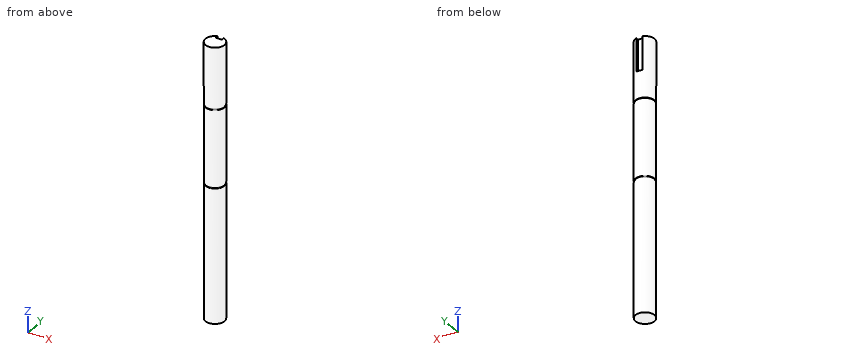
```python
from build123d import *

# Parameters (mm, degrees)
SKETCH_1_R          = 12.5
EXTRUDE_1_DEPTH     = 359
CUT_EXTRUDE_START   = -44
SKETCH_2_W          = 8
SKETCH_2_H          = 8.5
CUT_EXTRUDE_1_DEPTH = 44
SKETCH_3_W          = 1.4
SKETCH_3_H          = 2.395884976
SKETCH_3_H_2        = 2.262849939


with BuildPart() as part:
    # Эскиз1 → Бобышка-Вытянуть1 (new body)
    with BuildSketch(Plane.XY):
        Circle(SKETCH_1_R)
    extrude(amount=-EXTRUDE_1_DEPTH)

    # Эскиз2 → Вырез-Вытянуть1 (cut)
    with BuildSketch(Plane.XY.offset(CUT_EXTRUDE_START)):
        with Locations((0, 12.25)):
            Rectangle(SKETCH_2_W, SKETCH_2_H)
    extrude(amount=CUT_EXTRUDE_1_DEPTH, mode=Mode.SUBTRACT)

    # Эскиз3 → Вырез-Повернуть1 (revolve, cut)
    with BuildSketch(Plane(origin=(0, 0, 0), x_dir=(0, 0, -1), z_dir=(1, 0, 0))):
        with Locations((182.35, 12.947942488)):
            Rectangle(SKETCH_3_W, SKETCH_3_H)
        with Locations((80.55, 12.881424969)):
            Rectangle(SKETCH_3_W, SKETCH_3_H_2)
    revolve(axis=Axis((0, 0, 1000), (0, 0, -1)), mode=Mode.SUBTRACT)


solid = part.part
```
Here's how the part is built. I have some questions about the finished solid (model axes, mm). Coordinates: 2 decimals unless noted, no trailing zeros. Loops run counter-clockwise (first coordinate to the right, second up) from the corner with the lowest first, then second, coordinate; pieces in that order, holes last. Notation, with made-up numbers: (36, -13) - (51, -13) arc R24 ccw to (51, 16) - close; hole circle Ø7 at (53.25, -14.5). An arc over 180 degrees is marked (long way). Return JSON: item names as keys, results as strings. Group by question number.
Item 1: Will these pins go through, and if not, where does the flat tip stop? P1, Ø8, axis at x = -10, z = -150.5, coming from the +Y side; P2, Ø5, axis at y = -6.5, z = -282.5, coming from the +X side; P3, Ø1.2, axis at y = 9.5, z = -12, coming from the -X side.
Item 2: I need wall thicknesses on line 1 (Y direction, x = -0.75, z = -136); line 2 (X direction, y = 8.5, z = -31); line 3 (X direction, y = 2.25, z = -221.5). Which ranges of each line are inside material? Lowest first, please. Write a range as from..to.
Item 3: If we section it at B-B on y = -4.75: Write out the boundary of the cut face in (x, z).
Item 4: If we section it at C-C on z = -224: Write out the boundary of the cut face in (x, y), and give its area (3 significant figures).
Item 5: If we section it at A-A on x = 0: Write out the boundary of the cut face in (y, z).
Calculated:
{
 "1": {"P1": "stops at y = 10.97", "P2": "stops at x = 11.84", "P3": "stops at x = -8.78"},
 "2": {"line 1": "y = -12.48..12.48", "line 2": "x = -9.17..-4, 4..9.17", "line 3": "x = -12.3..12.3"},
 "3": {"outline": "(-11.56, -359) - (11.56, -359) - (11.56, -183.05) - (10.75, -183.05) - (10.75, -181.65) - (11.56, -181.65) - (11.56, -81.25) - (10.75, -81.25) - (10.75, -79.85) - (11.56, -79.85) - (11.56, 0) - (-11.56, 0) - (-11.56, -79.85) - (-10.75, -79.85) - (-10.75, -81.25) - (-11.56, -81.25) - (-11.56, -181.65) - (-10.75, -181.65) - (-10.75, -183.05) - (-11.56, -183.05) - close"},
 "4": {"outline": "circle Ø25 at (0, 0)", "area": "491 mm^2"},
 "5": {"outline": "(-12.5, -359) - (12.5, -359) - (12.5, -183.05) - (11.75, -183.05) - (11.75, -181.65) - (12.5, -181.65) - (12.5, -81.25) - (11.75, -81.25) - (11.75, -79.85) - (12.5, -79.85) - (12.5, -44) - (8, -44) - (8, 0) - (-12.5, 0) - (-12.5, -79.85) - (-11.75, -79.85) - (-11.75, -81.25) - (-12.5, -81.25) - (-12.5, -181.65) - (-11.75, -181.65) - (-11.75, -183.05) - (-12.5, -183.05) - close"}
}
